from build123d import *

# Parameters (mm, degrees)
SKETCH1_R           = 25
SKETCH1_R_2         = 1.5
BOSS_EXTRUDE1_DEPTH = 3
BOSS_EXTRUDE2_DEPTH = 40
SKETCH4_R           = 1.375
CUT_EXTRUDE1_DEPTH  = 7.5
CUT_EXTRUDE2_DEPTH  = 2.35


with BuildPart() as part:
    # Sketch1 → Boss-Extrude1 (new body)
    with BuildSketch(Plane(origin=(0, 0, 0), x_dir=(1, 0, 0), z_dir=(0, 1, 0))):
        with Locations(Location((0, 0, 0), (0, 0, 270))):
            Circle(SKETCH1_R)
        with Locations(Location((0, 20.5, 0), (0, 0, 270))):
            Circle(SKETCH1_R_2, mode=Mode.SUBTRACT)
        with Locations(Location((17.753520778, -10.25, 0), (0, 0, 270))):
            Circle(SKETCH1_R_2, mode=Mode.SUBTRACT)
        with Locations(Location((-17.753520778, -10.25, 0), (0, 0, 270))):
            Circle(SKETCH1_R_2, mode=Mode.SUBTRACT)
    extrude(amount=BOSS_EXTRUDE1_DEPTH)

    # Sketch3 → Boss-Extrude2 (add)
    with BuildSketch(Plane(origin=(0, 3, 0), x_dir=(1, 0, 0), z_dir=(0, 1, 0))):
        Polygon((-6.92820323, 0), (-3.464101615, -6), (3.464101615, -6), (6.92820323, 0), (3.464101615, 6), (-3.464101615, 6), align=None)
    extrude(amount=BOSS_EXTRUDE2_DEPTH)

    # Sketch4 → Cut-Extrude1 (cut)
    with BuildSketch(Plane(origin=(0, 43, 0), x_dir=(1, 0, 0), z_dir=(0, 1, 0))):
        with Locations(Location((0, 0, 0), (0, 0, 270))):
            Circle(SKETCH4_R)
    extrude(amount=-CUT_EXTRUDE1_DEPTH, mode=Mode.SUBTRACT)

    # Sketch5 → Cut-Extrude2 (cut)
    with BuildSketch(Plane(origin=(0, 3, 0), x_dir=(1, 0, 0), z_dir=(0, 1, 0))):
        Polygon((1.567505981, 23.215), (-1.567505981, 23.215), (-3.135011962, 20.5), (-1.567505981, 17.785), (1.567505981, 17.785), (3.135011962, 20.5), align=None)
        Polygon((19.321026758, -12.965), (20.888532739, -10.25), (19.321026758, -7.535), (16.186014797, -7.535), (14.618508816, -10.25), (16.186014797, -12.965), align=None)
        Polygon((-20.888532739, -10.25), (-19.321026758, -12.965), (-16.186014797, -12.965), (-14.618508816, -10.25), (-16.186014797, -7.535), (-19.321026758, -7.535), align=None)
    extrude(amount=-CUT_EXTRUDE2_DEPTH, mode=Mode.SUBTRACT)


solid = part.part
Design review of the part built by this model. Coordinates are the model's own, in mm. A direction names the side the tool comes from. Give positions to 0.01 mm unless a question says otherwise; leave off trailing zeros. Write each loop counter-clockwise with the first axis right and the second up, starting at its lowest first coordinate (ties: lowest second). Pieces come first, ordered by that corner, then holes. Notation, with made-up numbers: M 82,85.5 L 116,85.5 A23 ccw 116,105.5 Z; hole C -7,34.5 d9. An arc over 180 degrees is marked long. Return JSON: item names as keys, results as strings. Group by question number.
Item 1: Take a section at D-D (z = -11.5). Give the boundary of the cut face in (x, y), plus the area to 3 significant figures.
Item 2: Tool access review of faces 4 (the flat face through (-5.172, 22.72, -3.042)), 5 (the flat face through (0, 23, -6)), 6 (the flat face through (5.22, 22.72, -2.96)), 7 (the flat face through (-5, 3, 5)): name each direction out of +Z, -Z, +X, -X, +Y, -Y from which nothing blocks a thin tool from reaching the whole face with its end or side.
Item 3: Clearance check with flat-ended pins moving along their axes: pin 1 Ø2.5 at (x, y) = (-17.5, 1.5) entering from +Z; pin 2 Ø12 at (y, z) = (36.5, -15) entering from +X; pin 3 Ø10 at (x, y) = (-7, 20) entering from +Z; pin 4 Ø10 at (x, z) = (16, -9) entering from +Y. State where each tip first meets the part, or that it passes through.
Item 4: Take a section at A-A (x = 0). Give the boundary of the cut face in (y, z) (3 decimals), plus the area to 3 significant figures.
Item 5: Wall thickness on line 1 along Y through (x, z) = (-2, 13.5); line 2 along Z through (x, y) = (-2, 4.5); line 3 along X through (y, z) = (0.2, -20.5): over which ranges is each line inside the solid? List them lowest first.
Item 6: Take a section at B-B (y = 7.5). Give the boundary of the cut face in (x, z), plus the area to 3 significant figures.
Item 7: The part is to be moulded in two halves that separate along X. For faces 1 (the flat face through (0, 23, 6)), 2 (the flat face through (-16, 0.65, 9)), 3 (the flat face through (-5.22, 22.72, 2.96)), say which applies: pulls with the +X half, pulls with the -X half, needs draft (parallel to the pull), parting line crosses it, or undercut.
Item 8: Take a section at C-C (x = 17). Give the boundary of the cut face in (y, z) (3 decimals), plus the area to 3 significant figures.
Return value:
{
 "1": {"outline": "M -22.2,0 L 22.2,0 L 22.2,3 L -22.2,3 Z", "area": "133 mm2"},
 "2": {"face 4": "-Z, -X, +Y", "face 5": "-Z, +X, -X, +Y", "face 6": "-Z, +X, +Y", "face 7": "+Y"},
 "3": {"pin 1": "stops at z = 19", "pin 2": "passes through", "pin 3": "stops at z = 6", "pin 4": "stops at y = 3"},
 "4": {"outline": "M 0,-25 L 3,-25 L 3,-23.215 L 0.65,-23.215 L 0.65,-22 L 0,-22 Z; M 0,-19 L 0.65,-19 L 0.65,-17.785 L 3,-17.785 L 3,-6 L 43,-6 L 43,-1.375 L 35.5,-1.375 L 35.5,1.375 L 43,1.375 L 43,6 L 3,6 L 3,25 L 0,25 Z", "area": "595 mm2"},
 "5": {"line 1": "y = 0 to 3", "line 2": "z = -6 to 6", "line 3": "x = -14.31 to -1.5, 1.5 to 14.31"},
 "6": {"outline": "M -6.93,0 L -3.46,-6 L 3.46,-6 L 6.93,0 L 3.46,6 L -3.46,6 Z", "area": "125 mm2"},
 "7": {"face 1": "needs draft", "face 2": "undercut", "face 3": "pulls with the -X half"},
 "8": {"outline": "M 0,-18.33 L 3,-18.33 L 3,7.535 L 0.65,7.535 L 0.65,8.953 L 0,8.953 Z; M 0,11.547 L 0.65,11.547 L 0.65,12.965 L 3,12.965 L 3,18.33 L 0,18.33 Z", "area": "95.5 mm2"}
}
